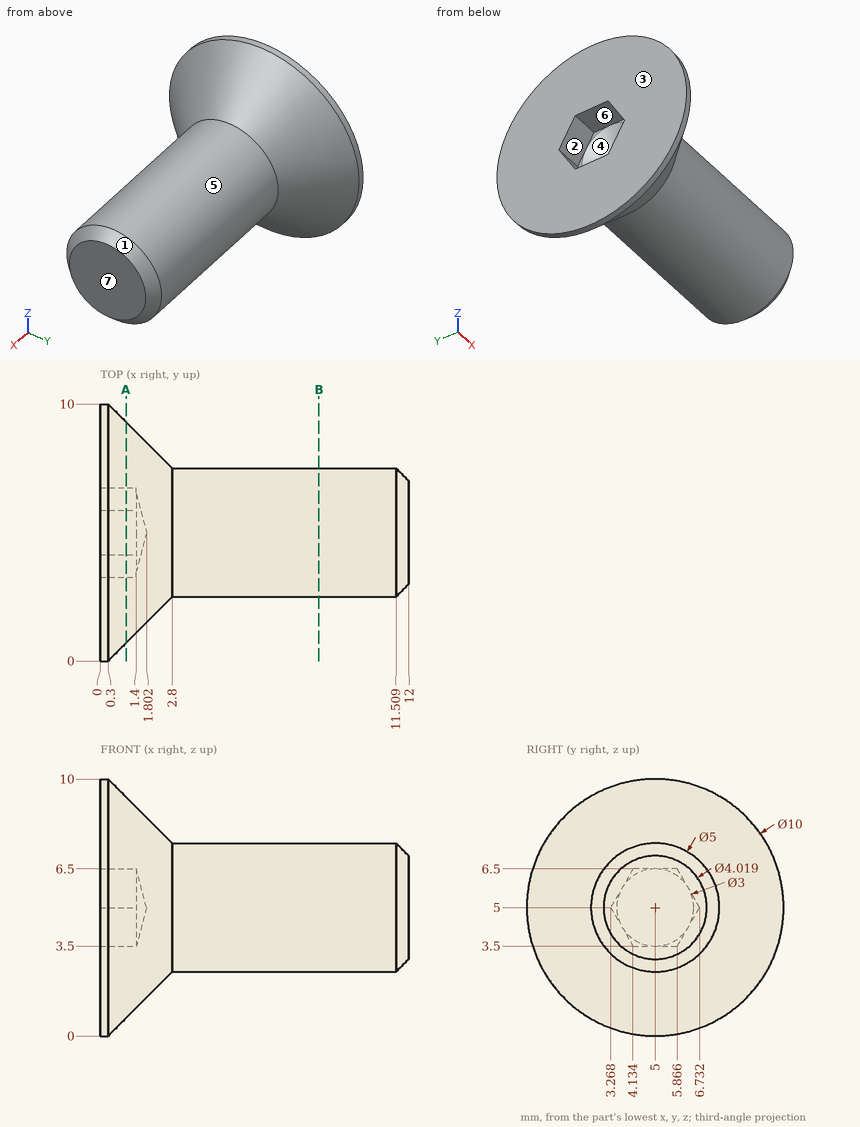
Geometry check sheet. Reference: drawing and pictorial views, mm from the part's lowest x, y, z. A direction names the side the tool comes from. Round coordinates to 2 decimals unless told otherwise and drop trailing zeros. Loops run counter-clockwise (first coordinate to the right, second up) from the corner with the lowest first, then second, coordinate; pieces in that order, holes last. Notation, with made-up numbers: (81, -14.75) - (118, -14.75) arc R29 ccw to (118, 13.25) - close; hole circle Ø9 at (12, 82.25). An arc over 180 degrees is marked (long way). Answer in a Markdown table with one row per item. Add a question column.
Q1. Tool access check on the marked faces 5, 6 and 7. Record the directions out of +Z, -Z, +X, -X, +Y, -Y that give a thin tool (end or side, any length) a straight path to the whole face; none if there is none.
Q2. Section check A-A on x = 1. Enter the section's corners in (y, z) (1 decimal), plus the area to 3 significant figures.
Q3. Material ranges on line 1 (Z direction, x = 10.75, y = 5); line 2 (Z direction, x = 4.25, y = 7); line 3 (Y direction, x = 0.75, z = 4.75) (1 decimal), recorded low to high.
Q4. Release check for a two-part mould opening along Z. For the marked faces 1, 2, 3 and 4 record: pulls with the +Z half, pulls with the -Z half, needs draft (parallel to the pull), parting line crosses it, or undercut.
Q5. Section check B-B on x = 8.5. Enter the section's corners in (y, z).
Q6. Gauge pin test, flat ends, axial feed: pin 1 (1.5 mm diameter, centred on x = 10.5, y = 3.5, fed in from -Z) (1 decimal); pin 2 (1 mm diameter, centred on x = 3, z = 7, fed in from -Y). Record the tip position at first contact, or that the pin passes through.
Found:
| question | item | result |
|---|---|---|
| 1 | face 5 | +X |
| 1 | face 6 | -X |
| 1 | face 7 | +Z, -Z, +X, +Y, -Y |
| 2 | outline | circle Ø8.6 at (5, 5); hole (3.3, 5) - (4.1, 3.5) - (5.9, 3.5) - (6.7, 5) - (5.9, 6.5) - (4.1, 6.5) - close |
| 2 | area | 50.3 mm² |
| 3 | line 1 | z = 2.5 to 7.5 |
| 3 | line 2 | z = 3.5 to 6.5 |
| 3 | line 3 | y = 0.5 to 3.4, 6.6 to 9.5 |
| 4 | face 1 | parting line crosses it |
| 4 | face 2 | undercut |
| 4 | face 3 | needs draft |
| 4 | face 4 | undercut |
| 5 | outline | circle Ø5 at (5, 5) |
| 6 | pin 1 | stops at z = 2.6 |
| 6 | pin 2 | stops at y = 2.9 |
